For this review, use the dimensioned drawing (mm, ordinates from the lowest corner) and the shaded views. Give positions to 0.01 mm unless a question says otherwise; leave off trailing zeros. Loops run counter-clockwise (first coordinate to the right, second up) from the corner with the lowest first, then second, coordinate; pieces in that order, holes last. Notation, with made-up numbers: M -28,59.5 L 20,59.5 A14 ccw 20,66.5 Z; hole C -5.5,30.25 d10. An arc over 180 degrees is marked long. Use CSV: the item, a comma, the result in double quotes.
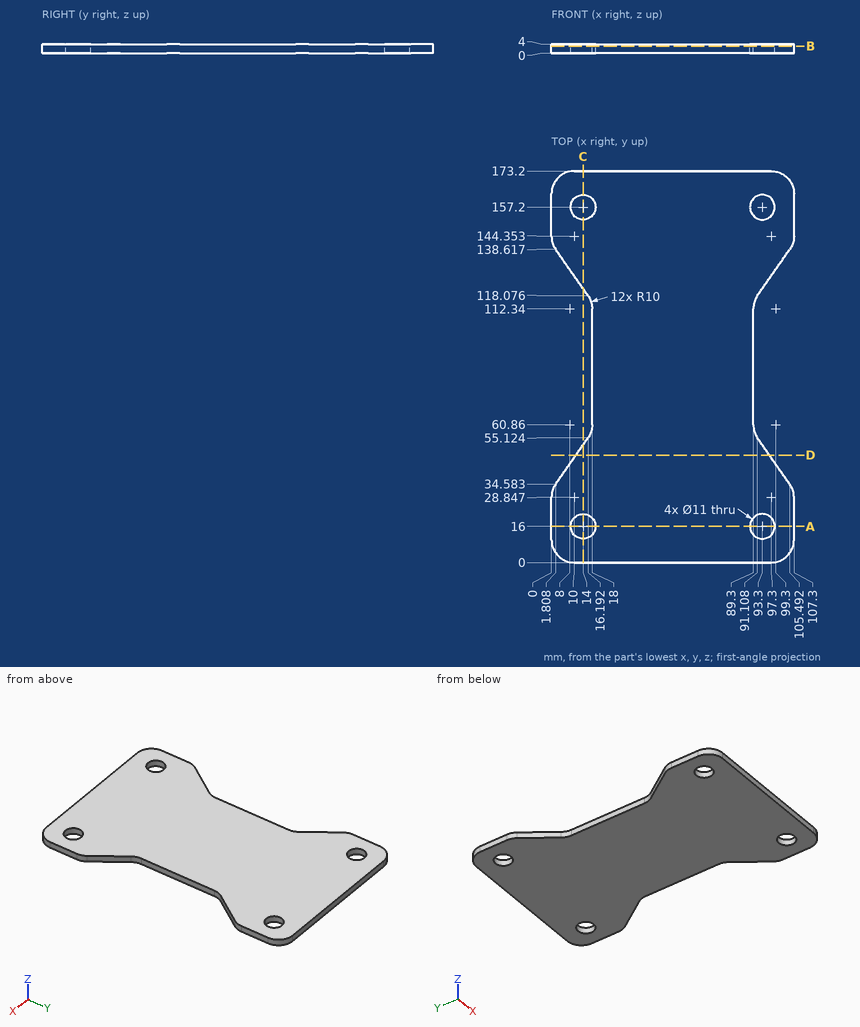
(1) We need section A-A on y = 16. State the section outline as (x, z) points.
A:
outline,"M 0,0 L 8.5,0 L 8.5,4 L 0,4 Z; M 19.5,0 L 87.8,0 L 87.8,4 L 19.5,4 Z; M 98.8,0 L 107.3,0 L 107.3,4 L 98.8,4 Z"
(2) We need section C-C on x = 14. State the section outline as (y, z) points (1 decimal), then the cut area to 3 significant figures.
A:
outline,"M 0,0 L 10.5,0 L 10.5,4 L 0,4 Z; M 21.5,0 L 52,0 L 52,4 L 21.5,4 Z; M 121.2,0 L 151.7,0 L 151.7,4 L 121.2,4 Z; M 162.7,0 L 173.2,0 L 173.2,4 L 162.7,4 Z"
area,"328 mm²"
(3) Clearance check with a flat-ended pin moving along its axis: P1, Ø2, axis at y = 142, z = 1.5, coming from the -X side. State where the tip first meets the part, or that it passes through.
A:
P1,"x = 0.09"
(4) We need section B-B on z = 3.1. State the section outline as (x, y) points.
A:
outline,"M 0,10 A10 ccw 10,0 L 97.3,0 A10 ccw 107.3,10 L 107.3,28.85 A10 ccw 105.49,34.58 L 91.11,55.12 A10 cw 89.3,60.86 L 89.3,112.34 A10 cw 91.11,118.08 L 105.49,138.62 A10 ccw 107.3,144.35 L 107.3,163.2 A10 ccw 97.3,173.2 L 10,173.2 A10 ccw 0,163.2 L 0,144.35 A10 ccw 1.81,138.62 L 16.19,118.08 A10 cw 18,112.34 L 18,60.86 A10 cw 16.19,55.12 L 1.81,34.58 A10 ccw 0,28.85 Z; hole C 14,16 d11; hole C 14,157.2 d11; hole C 93.3,16 d11; hole C 93.3,157.2 d11"
(5) Wall thickness on line 1 along X through (y, z) = (161, 1.75) (1 decimal); line 2 along X through (y, z) = (16, 2.7); line 3 along Y through (x, z) = (16.5, 2.6) (1 decimal): over which ranges is each line inside the solid? List them lowest first. Write a range as [from, to].
A:
line 1,"[0, 10], [18, 89.3], [97.3, 107.3]"
line 2,"[0, 8.5], [19.5, 87.8], [98.8, 107.3]"
line 3,"[0, 11.1], [20.9, 55.6], [117.6, 152.3], [162.1, 173.2]"
(6) We need section D-D on y = 47.5. State the section outline as (x, z) points.
A:
outline,"M 10.85,0 L 96.45,0 L 96.45,4 L 10.85,4 Z"
